Autodesk Inventor part; units mm, degrees
ref_plane "YZ Plane" through (0, 0, 0) normal (1, 0, 0) x (0, 1, 0)
sketch "スケッチ1" plane through (0, 0, 0) normal (0, 0, 1) x (1, 0, 0)
  arc A0 (0, 37.5) -> (0, -37.5) centre (0, 0) ccw
  line L0 (0, 37.5) -> (0, -37.5)
  dimension "d0" = 75
revolve "回転1" add sketch "スケッチ1" angle 360 about axis through (0, 37.5, 0) along (0, -1, 0)
sketch "スケッチ2" plane through (0, 0, 0) normal (0, 1, 0) x (-1, 0, 0)
  circle A0 centre (0, 0) radius 20
  dimension "d2" = 40
extrude "押し出し1" cut sketch "スケッチ2" along normal mid plane 100
sketch "スケッチ3" plane through (0, 0, 0) normal (0, 0, 1) x (1, 0, 0)
  circle A0 centre (0, 0) radius 25
  dimension "d5" = 50
extrude "押し出し2" add sketch "スケッチ3" against normal blind 50
properties part number "LowerarmP"
The listing builds one solid part. Answer for the finished solid, in the listing's coordinates (mm). A direction names the side the tool comes from. Give positions to 0.01 mm unless a question says otherwise; leave off trailing zeros. Write each loop counter-clockwise with the first axis right and the second up, starting at its lowest first coordinate (ties: lowest second). Pieces come first, ordered by that corner, then holes.
1) Find the intervals of material crossed by L1, parallel to Z at x = -1, y = -20; L2, parallel to Z at x = -4.5, y = -5.5; L3, parallel to X at y = 25, z = 4.5, in increasing order.
2) Given P1, Ø10, axis at x = -17, z = 28.5, coming from the -Y side; P2, Ø8, axis at x = -26, z = 2.5, coming from the -Y side; P3, Ø4, axis at y = 25, z = -30.5, coming from the -X side, each flat-ended and moving along its own axis, determine where each tip first touches the part or whether it passes through.
3) Section C-C (z = -3) is taken. Write down the section's boundary in (x, y).
4) Section D-D (z = 8) is taken. Write down the section's boundary in (x, y).
5) A tool of negligible diameter and unlimited length cuts with its end or side. For faces 1 (the face through (0, 0, 0)), 2 (the face through (23.846, 7.509, -38.821)), from which of +Z, -Z, +X, -X, +Y, -Y can it reach the whole face along a straight path? Write none if from no direction.
6) Section B-B (y = 0) is taken. Write down the section's boundary in (x, z), and give its area (3 significant figures).
7) For a pull along Z with two mould halves and no side action, classify faces 3 (the face through (0, 0, -50)), 4 (the face through (0, 25, -8)) as pulls with the +Z half, pulls with the -Z half, needs draft (parallel to the pull), parting line crosses it, or undercut.
8) Section A-A (x = 0) is taken. Write down the section's boundary in (y, z).
Response:
1. L1: z = -50 to 0, 19.97 to 31.71
1. L2: z = -50 to 0, 19.49 to 36.82
1. L3: x = -27.59 to -19.49, 19.49 to 27.59
2. P1: stops at y = -24.74
2. P2: stops at y = -30.28
2. P3: stops at x = -9.8
3. outline: (-19.77, -31.72) - (-19.77, -15.3) arc R25 ccw to (19.77, -15.3) - (19.77, -31.72) arc R37.38 ccw to (19.77, 31.72) - (19.77, 15.3) arc R25 ccw to (-19.77, 15.3) - (-19.77, 31.72) arc R37.38 ccw to start
4. outline: (-18.33, -31.72) - (-18.33, 31.72) arc R36.64 ccw to start; (18.33, -31.72) arc R36.64 ccw to (18.33, 31.72) - close
5. face 1: +Y, -Y
5. face 2: -Z
6. outline: (-25, -50) - (25, -50) - (25, -27.95) arc R37.5 ccw (long way) to (-25, -27.95) - close; hole (-20, 0) - (20, 0) arc R20 ccw to start
6. area: 4,560 mm2
7. face 3: pulls with the -Z half
7. face 4: undercut
8. outline: (-31.72, -20) arc R37.5 ccw to (-25, -27.95) - (-25, -50) - (25, -50) - (25, -27.95) arc R37.5 ccw to (31.72, -20) - (25, -20) - (25, 0) - (-25, 0) - (-25, -20) - close; (-31.72, 20) - (31.72, 20) arc R37.5 ccw to start
